Model file for the job. Use its own axes, mm. Give positions to 0.01 mm unless a question says otherwise; leave off trailing zeros. Order: outer loops, then holes, each group sorted by start corner. A loop starts at its lowest first (then second) coordinate and runs counter-clockwise, first axis right, second up. Notation, with made-up numbers: (40.5, -38.75) -> (57.5, -38.75) arc R15 cw to (57.5, -34.75) -> close; hole circle Ø6 at (54.5, -38). An arc over 180 degrees is marked (long way). Use CSV: the item, a comma, the result in double quotes. Start each with the question number.
1. Drop flat-ended pins along their axis: pin 1 (1.5 mm diameter, centred on x = 523, y = 14.5, fed in from +Z); pin 2 (10 mm diameter, centred on y = 2.5, z = -48, fed in from -X); pin 3 (15.5 mm diameter, centred on x = 21, z = 73.5, fed in from +Y). Give the stop position or say it passes through.
2. Wall check: line 1 (Y direction, x = 1042, z = 74.5); line 2 (Z direction, x = 189.5, y = -6.5); line 3 (X direction, y = -17, z = 36). Give the ranges that are in metal, low to high. Write a range as from..to.
3. Cut at A-A on x = 985. List the corners of the cut face in (y, z).
```python
from build123d import *

# Parameters (mm, degrees)
F1_W     = 40
F1_H     = 33
F1_W_2   = 8
F1_H_2   = 14
F3_DEPTH = 1240
F2_W     = 80
F2_H     = 100
F4_DEPTH = 25


with BuildPart() as f3:
    # F1 (on Right) → F3 (new body, symmetric)
    with BuildSketch(Plane.YZ):
        Polygon((20, 33), (20, 63), (17, 66), (12, 66), (12, 80), (4, 80), (4, 66), (-4, 66), (-4, 80), (-12, 80), (-12, 66), (-17, 66), (-20, 63), (-20, 33), align=None)
        with Locations((0, 16.5)):
            Rectangle(F1_W, F1_H)
        with Locations((0, -16.5)):
            Rectangle(F1_W, F1_H)
        Polygon((20, -52), (20, -33), (-20, -33), (-20, -52), (-12, -52), (-4, -52), (4, -52), (12, -52), align=None)
        Polygon((-12, -52), (-20, -52), (-20, -63), (-17, -66), (-12, -66), align=None)
        with Locations((0, -59)):
            Rectangle(F1_W_2, F1_H_2)
        Polygon((20, -63), (20, -52), (12, -52), (12, -66), (17, -66), align=None)
    extrude(amount=F3_DEPTH, both=True)

    # F2 (on Front) → F4 (cut, symmetric)
    with BuildSketch(Plane.XZ):
        with Locations((-1240, 83)):
            Rectangle(F2_W, F2_H)
        with Locations((-1240, -83)):
            Rectangle(F2_W, F2_H)
    extrude(amount=F4_DEPTH, both=True, mode=Mode.SUBTRACT)


solid = f3.part
```
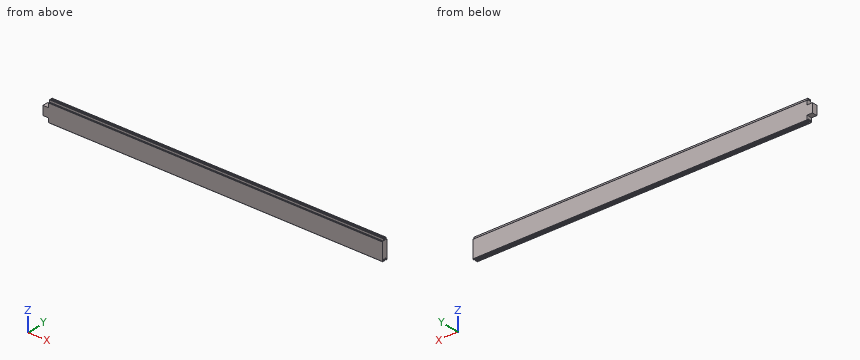
Verdict:
1,pin 1,"z = 66"
1,pin 2,"x = -1200"
1,pin 3,"y = 17.25"
2,line 1,"-12..-4, 4..12"
2,line 2,"-52..80"
2,line 3,"-1200..1240"
3,outline,"(-20, -63) -> (-17, -66) -> (-12, -66) -> (-12, -52) -> (-4, -52) -> (-4, -66) -> (4, -66) -> (4, -52) -> (12, -52) -> (12, -66) -> (17, -66) -> (20, -63) -> (20, 63) -> (17, 66) -> (12, 66) -> (12, 80) -> (4, 80) -> (4, 66) -> (-4, 66) -> (-4, 80) -> (-12, 80) -> (-12, 66) -> (-17, 66) -> (-20, 63) -> close"
